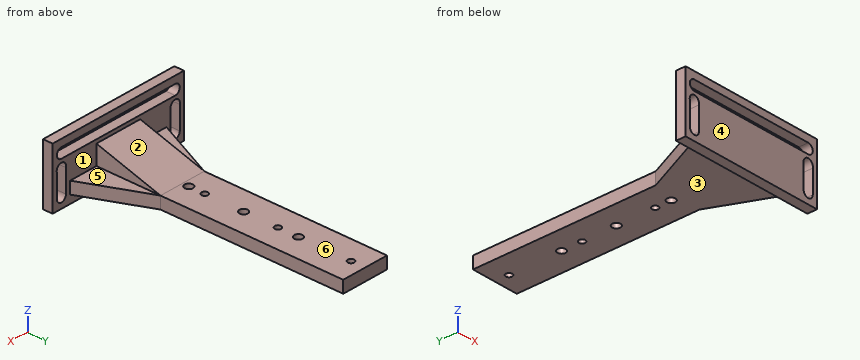
from build123d import *

# Parameters (mm, degrees)
SKETCH_1_W                = 90
SKETCH_1_H                = 90
EXTRUDE_1_DEPTH           = 6
SKETCH_2_W                = 30
SKETCH_2_H                = 40
EXTRUDE_2_DEPTH           = 160
EXTRUDE_3_DEPTH           = 20
SKETCH_8_R                = 3.1
CUT_EXTRUDE_2_DEPTH       = 6
EXTRUDE_4_DEPTH           = 15
CUT_EXTRUDE_4_DEPTH       = 173.191753577
CUT_EXTRUDE_4_DEPTH_BACK  = 173.191753577
SKETCH_17_W               = 25
SKETCH_17_H               = 154
SKETCH_21_W               = 15
SKETCH_21_H               = 6
CUT_EXTRUDE_8_DEPTH       = 173.191753577
SKETCH_23_W               = 78
SKETCH_23_H               = 6.2
CUT_EXTRUDE_9_DEPTH       = 173.191753577
MIRROR_14_COPY_1_SKETCH_R = 3.1
MIRROR_14_COPY_1_DEPTH    = 6
SKETCH_25_W               = 6.229282002
SKETCH_25_H               = 15
CUT_EXTRUDE_10_DEPTH      = 173.191753577
SKETCH_26_R               = 3.114641001
CUT_EXTRUDE_11_DEPTH      = 173.191753577
SKETCH_27_R               = 3.202321727
CUT_EXTRUDE_12_DEPTH      = 173.191753577
CUT_EXTRUDE_13_DEPTH      = 173.191753577
SKETCH_29_W               = 45
SKETCH_29_H               = 7.5
CUT_EXTRUDE_14_DEPTH      = 173.191753577
SKETCH_30_W               = 5
SKETCH_30_H               = 40
CUT_EXTRUDE_15_DEPTH      = 173.191753577
SKETCH_31_R               = 2
CUT_EXTRUDE_16_DEPTH      = 173.191753577
PATTERN_LINEAR_2_COUNT    = 3
PATTERN_LINEAR_2_PITCH    = 45.6
SKETCH_32_R               = 2.6
CUT_EXTRUDE_17_DEPTH      = 173.191753577
PATTERN_LINEAR_3_COUNT    = 3
PATTERN_LINEAR_3_PITCH    = 34.2


with BuildPart() as part:
    # 草图1 → 凸台-拉伸1 (new body)
    with BuildSketch(Plane(origin=(0, 0, 0), x_dir=(1, 0, 0), z_dir=(0, 1, 0))):
        Rectangle(SKETCH_1_W, SKETCH_1_H)
    extrude(amount=EXTRUDE_1_DEPTH)

    # 草图2 → 凸台-拉伸2 (add)
    with BuildSketch(Plane(origin=(0, 0, 0), x_dir=(1, 0, 0), z_dir=(0, 1, 0))):
        Rectangle(SKETCH_2_W, SKETCH_2_H)
    extrude(amount=EXTRUDE_2_DEPTH)

    # 草图7 → 凸台-拉伸3 (add)
    with BuildSketch(Plane.XY):
        Polygon((-15, 46), (-33, 6), (-15, 6), align=None)
    extrude_3 = extrude(amount=EXTRUDE_3_DEPTH)

    # 草图8 → 切除-拉伸2 (cut)
    with BuildSketch(Plane(origin=(0, 0, 0), x_dir=(1, 0, 0), z_dir=(0, 1, 0))):
        with Locations(Location((-39, 37.4, 0), (0, 0, 90))):
            Circle(SKETCH_8_R)
    cut_extrude_2 = extrude(amount=CUT_EXTRUDE_2_DEPTH, mode=Mode.SUBTRACT)

    # 草图15 → 凸台-拉伸4 (add, symmetric)
    with BuildSketch(Plane(origin=(0, 0, 0), x_dir=(0, 0, -1), z_dir=(1, 0, 0))):
        Polygon((-20, 46), (-20, 6), (-32, 6), align=None)
    extrude_4 = extrude(amount=EXTRUDE_4_DEPTH, both=True)

    # 镜向11: 凸台-拉伸4 across plane
    add(extrude_4.mirror(Plane.XY))

    # 草图17 → 切除-拉伸4 (cut, two sides: drawn at the far end of the back side and taken through both)
    with BuildSketch(Plane(origin=(0, 0, 0), x_dir=(0, 0, -1), z_dir=(1, 0, 0)).offset(-CUT_EXTRUDE_4_DEPTH_BACK)):
        with Locations((0, 83)):
            Rectangle(SKETCH_17_W, SKETCH_17_H)
    extrude(amount=CUT_EXTRUDE_4_DEPTH + CUT_EXTRUDE_4_DEPTH_BACK, mode=Mode.SUBTRACT)

    # 草图21 → 切除-拉伸8 (cut, through all)
    with BuildSketch(Plane(origin=(0, 0, 0), x_dir=(0, 0, -1), z_dir=(1, 0, 0))):
        with Locations((0, 3)):
            Rectangle(SKETCH_21_W, SKETCH_21_H)
    extrude(amount=-CUT_EXTRUDE_8_DEPTH, mode=Mode.SUBTRACT)

    # 镜向12: 切除-拉伸2 across plane
    add(cut_extrude_2.mirror(Plane(origin=(0, 0, 0), x_dir=(0, 0, 1), z_dir=(1, 0, 0))), mode=Mode.SUBTRACT)

    # 草图23 → 切除-拉伸9 (cut, through all)
    with BuildSketch(Plane(origin=(0, 0, 0), x_dir=(1, 0, 0), z_dir=(0, 1, 0))):
        with Locations((0, 37.4)):
            Rectangle(SKETCH_23_W, SKETCH_23_H)
    cut_extrude_9 = extrude(amount=CUT_EXTRUDE_9_DEPTH, mode=Mode.SUBTRACT)

    # 镜向13: 切除-拉伸9 across plane
    add(cut_extrude_9.mirror(Plane.XY), mode=Mode.SUBTRACT)

    # 镜向14: 切除-拉伸2 across plane
    add(cut_extrude_2.mirror(Plane.XY), mode=Mode.SUBTRACT)

    # 镜向14 copy 1 sketch → 镜向14 copy 1 (cut)
    with BuildSketch(Plane(origin=(0, 0, 0), x_dir=(-1, 0, 0), z_dir=(0, 1, 0))):
        with Locations(Location((-39, 37.4, 0), (0, 0, 90))):
            Circle(MIRROR_14_COPY_1_SKETCH_R)
    extrude(amount=MIRROR_14_COPY_1_DEPTH, mode=Mode.SUBTRACT)

    # 草图25 → 切除-拉伸10 (cut, through all)
    with BuildSketch(Plane(origin=(0, 0, 0), x_dir=(1, 0, 0), z_dir=(0, 1, 0))):
        with Locations((38.985358999, -21.5)):
            Rectangle(SKETCH_25_W, SKETCH_25_H)
    cut_extrude_10 = extrude(amount=CUT_EXTRUDE_10_DEPTH, mode=Mode.SUBTRACT)

    # 草图26 → 切除-拉伸11 (cut, through all)
    with BuildSketch(Plane(origin=(0, 0, 0), x_dir=(1, 0, 0), z_dir=(0, 1, 0))):
        with Locations((38.985358999, -14)):
            Circle(SKETCH_26_R)
    cut_extrude_11 = extrude(amount=CUT_EXTRUDE_11_DEPTH, mode=Mode.SUBTRACT)

    # 草图27 → 切除-拉伸12 (cut, through all)
    with BuildSketch(Plane(origin=(0, 0, 0), x_dir=(1, 0, 0), z_dir=(0, 1, 0))):
        with Locations((38.985358999, -29)):
            Circle(SKETCH_27_R)
    cut_extrude_12 = extrude(amount=CUT_EXTRUDE_12_DEPTH, mode=Mode.SUBTRACT)

    # 镜向15: 切除-拉伸10 across plane
    add(cut_extrude_10.mirror(Plane(origin=(0, 0, 0), x_dir=(0, 0, 1), z_dir=(1, 0, 0))), mode=Mode.SUBTRACT)

    # 镜向16: 切除-拉伸11 across plane
    add(cut_extrude_11.mirror(Plane(origin=(0, 0, 0), x_dir=(0, 0, 1), z_dir=(1, 0, 0))), mode=Mode.SUBTRACT)

    # 镜向17: 切除-拉伸12 across plane
    add(cut_extrude_12.mirror(Plane(origin=(0, 0, 0), x_dir=(0, 0, 1), z_dir=(1, 0, 0))), mode=Mode.SUBTRACT)

    # 镜向23: 凸台-拉伸3 across plane
    add(extrude_3.mirror(Plane(origin=(0, 0, 0), x_dir=(0, 0, 1), z_dir=(1, 0, 0))))

    # 草图28 → 切除-拉伸13 (cut, through all)
    with BuildSketch(Plane(origin=(0, 0, 0), x_dir=(1, 0, 0), z_dir=(0, 1, 0))):
        Polygon((45, 0), (0, 0), (0, 7.5), (-45, 7.5), (-45, 45), (45, 45), align=None)
    extrude(amount=CUT_EXTRUDE_13_DEPTH, mode=Mode.SUBTRACT)

    # 草图29 → 切除-拉伸14 (cut, through all)
    with BuildSketch(Plane(origin=(0, 0, 0), x_dir=(1, 0, 0), z_dir=(0, 1, 0))):
        with Locations((22.5, -3.75)):
            Rectangle(SKETCH_29_W, SKETCH_29_H)
    extrude(amount=CUT_EXTRUDE_14_DEPTH, mode=Mode.SUBTRACT)

    # 草图30 → 切除-拉伸15 (cut, through all)
    with BuildSketch(Plane(origin=(0, 0, 0), x_dir=(0, 0, -1), z_dir=(1, 0, 0))):
        with Locations((-10, 26)):
            Rectangle(SKETCH_30_W, SKETCH_30_H)
    extrude(amount=CUT_EXTRUDE_15_DEPTH, mode=Mode.SUBTRACT)

    # 草图31 → 切除-拉伸16 (cut, through all)
    with BuildSketch(Plane.XY):
        with Locations(Location((0, 60, 0), (0, 0, 180))):
            Circle(SKETCH_31_R)
    cut_extrude_16 = extrude(amount=CUT_EXTRUDE_16_DEPTH, mode=Mode.SUBTRACT)

    # 阵列(线性)2: 切除-拉伸16 ×3
    with Locations(*[(0, i * PATTERN_LINEAR_2_PITCH, 0) for i in range(1, PATTERN_LINEAR_2_COUNT)]):
        add(cut_extrude_16, mode=Mode.SUBTRACT)

    # 草图32 → 切除-拉伸17 (cut, through all)
    with BuildSketch(Plane.XY):
        with Locations(Location((0, 50, 0), (0, 0, 180))):
            Circle(SKETCH_32_R)
    cut_extrude_17 = extrude(amount=CUT_EXTRUDE_17_DEPTH, mode=Mode.SUBTRACT)

    # 阵列(线性)3: 切除-拉伸17 ×3
    with Locations(*[(0, i * PATTERN_LINEAR_3_PITCH, 0) for i in range(1, PATTERN_LINEAR_3_COUNT)]):
        add(cut_extrude_17, mode=Mode.SUBTRACT)


solid = part.part
Model file for the job. Use its own axes, mm. Face numbers are marked on the shaded views. A direction names the side the tool comes from. Give positions to 0.01 mm unless a question says otherwise; leave off trailing zeros. Loops run counter-clockwise (first coordinate to the right, second up) from the corner with the lowest first, then second, coordinate; pieces in that order, holes last.
1) Saw through at B-B (x = 23). Write the cut outline in (y, z).
2) Wall check: line 1 (X direction, y = 4.65, z = 29); line 2 (X direction, y = 151.2, z = 17); line 3 (X direction, y = 59.5, z = 19). Give the ranges that are in metal, low to high.
3) Saw through at C-C (z = 39). Write the cut outline in (x, y), plus the area to 3 significant figures.
4) Pull direction Z, two halves, no side cores. Call the marked faces 1, 2 and 3: +Z half, -Z half, draft (parallel to the pull), parting line (faces both ways), or undercut.
5) Tool access for the marked faces 4, 5 and 6: list every direction of +Z, -Z, +X, -X, +Y, -Y with a clear straight run to the whole face (end or side of a thin tool).
6) Saw through at D-D (y = 27). Write the cut outline in (x, z).
7) Saw through at A-A (y = 84.2). Write the cut outline in (x, z), plus the area to 3 significant figures.
8) Flat gauge pins, fed straight in: pin 1 Ø1 at (x, y) = (2, 72.5) entering from +Z; pin 2 Ø2 at (x, y) = (-14, 127) entering from -Z; pin 3 Ø4 at (x, y) = (0, 118.4) entering from +Z; pin 4 Ø8 at (y, z) = (128, 17) entering from -X. Where does each tip first touch, or does it go through?
Answer block:
1. outline: (0, 7.5) - (6, 7.5) - (6, 12.5) - (28.22, 12.5) - (28.22, 20) - (6, 20) - (6, 34.3) - (0, 34.3) - close; (0, 40.5) - (6, 40.5) - (6, 45) - (0, 45) - close
2. line 1: x = -45 to -42.19, -35.78 to 35.78, 42.19 to 45
2. line 2: x = -15 to -2, 2 to 15
2. line 3: x = -15 to -1.94, 1.94 to 15
3. outline: (-45, 0) - (-41.66, 0) - (-41.66, 6) - (-45, 6) - close; (41.66, 0) - (45, 0) - (45, 6) - (41.66, 6) - close
3. area: 40.1 mm2
4. face 1: draft
4. face 2: +Z half
4. face 3: -Z half
5. face 4: +Z, -Z, +X, -X, -Y
5. face 5: +Z, +X, +Y
5. face 6: +Z, +X, -X, +Y
6. outline: (-23.55, 12.5) - (23.55, 12.5) - (23.55, 20) - (15, 20) - (15, 25.7) - (-15, 25.7) - (-15, 20) - (-23.55, 20) - close
7. outline: (-15, 12.5) - (-2.6, 12.5) - (-2.6, 20) - (-15, 20) - close; (2.6, 12.5) - (15, 12.5) - (15, 20) - (2.6, 20) - close
7. area: 186 mm2
8. pin 1: stops at z = 20
8. pin 2: stops at z = 12.5
8. pin 3: passes through
8. pin 4: stops at x = -15
